For this review, take the finished solid that the model builds, in its own axes (mm). Face numbers are marked on the shaded views. A direction names the side the tool comes from. Round coordinates to 2 decimals unless told otherwise and drop trailing zeros. Write each loop counter-clockwise with the first axis right and the second up, starting at its lowest first coordinate (ties: lowest second). Pieces come first, ordered by that corner, then holes. Notation, with made-up numbers: (-11.5, 70) -> (-7.5, 70) arc R15 ccw to (-7.5, 80) -> close; hole circle Ø5 at (-15, 48.5). An arc over 180 degrees is marked (long way). Answer as CSV lines item,"result". Start each with the question number.
Item 1: Take a section at B-B on z = -290. Give the boundary of the cut face in (x, y), then the cut area to 3 significant figures.
Item 2: Take a section at A-A on z = -270. Give the boundary of the cut face in (x, y), then the cut area to 3 significant figures.
Item 3: Machinability: for the marked faces 1 and 2, which of the approach directions +Z, -Z, +X, -X, +Y, -Y give a long, thin tool a straight path to every point of the face, cutting with its end or side? Answer none if there is none.
Item 4: For pin 1 Ø5.5 at (x, y) = (-22.11, 35.16) entering from +Z; pin 2 Ø10 at (y, z) = (-65, -343.5) entering from -X; pin 3 Ø1.5 at (y, z) = (42.5, -337.5) entering from -X, all flat-tipped, find the tip position at first contact; note any pin that passes through.
Item 5: Wall thickness on probe 1 along Y at (x, z) = (-30.5, -297); probe 2 along Z at (x, y) = (45.5, -2); probe 3 along Y at (x, z) = (69.5, -329.5): over which ranges is each line inside the solid? List them lowest first. Write a range as from..to.
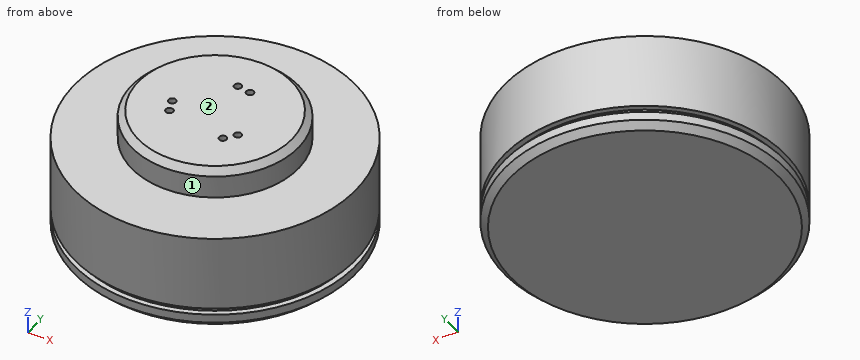
```python
from build123d import *

# Parameters (mm, degrees)
BOSS_EXTRUDE1_START        = -120.0001
BOSS_EXTRUDE1_OUTLINE_R    = 130
BOSS_EXTRUDE1_DEPTH        = 90.0001
SKETCH2_R                  = 130
SKETCH2_R_2                = 125
CUT_EXTRUDE1_DEPTH         = 6
SKETCH3_R                  = 77
BOSS_EXTRUDE2_DEPTH        = 26.9999
M8X1_25_TAPPED_HOLE1_D     = 6.8
M8X1_25_TAPPED_HOLE1_DEPTH = 19.75
M8X1_25_TAPPED_HOLE1_TIP   = 2.042926105
CHAMFER1_SIZE              = 6
CHAMFER2_SIZE              = 6


# Read off the part's stored shape, not the designer's step: Boss-Extrude1
with BuildPart() as part:
    # Boss-Extrude1 outline → Boss-Extrude1 (new body)
    with BuildSketch(Plane(origin=(0, 0, -406.611081847), x_dir=(-1, 0, 0), z_dir=(0, 0, -1)).offset(BOSS_EXTRUDE1_START)):
        with Locations((34.426276825, 1.328199188)):
            Circle(BOSS_EXTRUDE1_OUTLINE_R)
    extrude(amount=BOSS_EXTRUDE1_DEPTH)

    # Sketch2 → Cut-Extrude1 (cut)
    with BuildSketch(Plane(origin=(0, 0, -356.611081847), x_dir=(-1, 0, 0), z_dir=(0, 0, -1))):
        with Locations((34.426276825, 1.328199188)):
            Circle(SKETCH2_R)
        with Locations((34.426276825, 1.328199188)):
            Circle(SKETCH2_R_2, mode=Mode.SUBTRACT)
    extrude(amount=CUT_EXTRUDE1_DEPTH, mode=Mode.SUBTRACT)

    # Sketch3 → Boss-Extrude2 (add)
    with BuildSketch(Plane.XY.offset(-286.610981847)):
        with Locations((-34.426276825, 1.328199188)):
            Circle(SKETCH3_R)
    extrude(amount=BOSS_EXTRUDE2_DEPTH)

    # M8x1.25 Tapped Hole1
    with Locations(Plane.XY.offset(-259.611081847)):
        with Locations((-34.426276825, 37.328199188), (-22.113551665, 35.157133536), (-3.249362288, -16.671800812), (-11.285922876, -26.249400764), (-65.603191361, -16.671800812), (-69.879355933, -4.923135208)):
            Hole(M8X1_25_TAPPED_HOLE1_D / 2, depth=M8X1_25_TAPPED_HOLE1_DEPTH)
            with Locations((0, 0, -(M8X1_25_TAPPED_HOLE1_DEPTH + M8X1_25_TAPPED_HOLE1_TIP / 2))):  # 118° drill point
                Cone(0, M8X1_25_TAPPED_HOLE1_D / 2, M8X1_25_TAPPED_HOLE1_TIP, mode=Mode.SUBTRACT)

    # Chamfer1
    chamfer1_edges = [part.edges().sort_by_distance(p)[0] for p in [
        (-111.426276825, 1.328199188, -259.611081847),
    ]]
    chamfer(chamfer1_edges, length=CHAMFER1_SIZE)

    # Chamfer2
    chamfer2_edges = [part.edges().sort_by_distance(p)[0] for p in [
        (95.573723175, 1.328199188, -376.611081847),
    ]]
    chamfer(chamfer2_edges, length=CHAMFER2_SIZE)


solid = part.part
```
Output values:
1,outline,"circle Ø260 at (-34.43, 1.33)"
1,area,"53,100 mm^2"
2,outline,"circle Ø154 at (-34.43, 1.33); hole circle Ø6.8 at (-69.88, -4.92); hole circle Ø6.8 at (-65.6, -16.67); hole circle Ø6.8 at (-34.43, 37.33); hole circle Ø6.8 at (-22.11, 35.16); hole circle Ø6.8 at (-11.29, -26.25); hole circle Ø6.8 at (-3.25, -16.67)"
2,area,"18,400 mm^2"
3,face 1,"+Z"
3,face 2,"+Z, +X, -X, +Y, -Y"
4,pin 1,"stops at z = -279.75"
4,pin 2,"stops at x = -149.05"
4,pin 3,"stops at x = -157.98"
5,probe 1,"y = -128.61..131.27"
5,probe 2,"z = -376.61..-286.61"
5,probe 3,"y = -76.77..79.43"
